Source: CAD feature listing. Evaluate the final solid. Frame: model axes, mm. Face numbers are marked on the shaded views. Give positions to 0.01 mm unless a question says otherwise; leave off trailing zeros. Loops run counter-clockwise (first coordinate to the right, second up) from the corner with the lowest first, then second, coordinate; pieces in that order, holes last. Notation, with made-up numbers: M -16,-36 L 3,-36 A10 cw 3,-23 Z; hole C 45.25,61 d9. An arc over 180 degrees is marked long. Put each result on its own line as item: value.
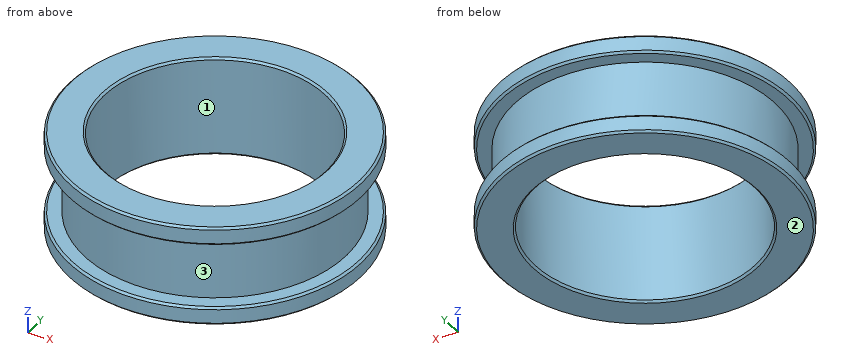
Autodesk Inventor part; units mm, degrees
ref_plane "Work Plane1" through (0, 0, 2.5) normal (0, 0, 1) x (1, 0, 0)
ref_plane "YZ Plane" through (0, 0, 0) normal (1, 0, 0) x (0, 1, 0)
ref_plane "XZ Plane" through (0, 0, 0) normal (0, 1, 0) x (-1, 0, 0)
sketch "Sketch1" plane through (0, 0, 0) normal (0, 0, 1) x (1, 0, 0)
  circle A0 centre (0, 0) radius 7.25
  dimension "d0" = 14.5
extrude "Extrusion1" add sketch "Sketch1" along normal blind 5
sketch "Sketch2" plane through (0, 0, 5) normal (0, 0, 1) x (1, 0, 0)
  circle A0 centre (0, 0) radius 5.5
  dimension "d3" = 11
extrude "Extrusion2" cut sketch "Sketch2" against normal through all
ref_plane "Work Plane1" through (0, 0, 2.5) normal (0, 0, 1) x (1, 0, 0)
sketch "Sketch3" plane through (0, 0, 2.5) normal (0, 0, 1) x (1, 0, 0)
  circle A0 centre (0, 0) radius 5.5
  circle A1 centre (0, 0) radius 6.5
  circle A2 centre (0, 0) radius 7.25
  dimension "d6" = 13
extrude "Extrusion3" cut sketch "Sketch3" along normal mid plane 3.2 contours A2
chamfer "Chamfer1" distance 0.1 angle 45 6 edges at (-7.25, 0, 4.1) (-7.25, 0, 0.9) (-7.25, 0, 0) (-7.25, 0, 5) (-5.5, 0, 0) (-5.5, 0, 5)
properties part number "roller" material "Aluminum 3004-H38"
1. Section query C-C (z = 4.45). Output: boundary loops of the cut face in (x, y), plus the area to 3 significant figures.
Found:
outline: C 0,0 d14.5; hole C 0,0 d11
area: 70.1 mm^2
2. Material intervals for line 1 (Y direction, x = 0, z = 4.55); line 2 (Y direction, x = 0, z = 3); line 3 (X direction, y = 4.5, z = 4), sorted ascending. Write a range as from..to.
Found:
line 1: -7.25..-5.5, 5.5..7.25
line 2: -6.5..-5.5, 5.5..6.5
line 3: -4.69..-3.16, 3.16..4.69
3. Contact query for flat-ended pins moving along their axis: P1, Ø1, axis at x = 4.5, z = 4.5, coming from the +Y side; P2, Ø1.5, axis at x = -1.5, z = 1, coming from the -Y side; P3, Ø2, axis at y = -2.5, z = 3, coming from the -X side. Output: stop coordinate, or through.
Found:
P1: y = 6.05
P2: y = -7.21
P3: x = -6.32
4. Section query D-D (z = 2.55). Output: boundary loops of the cut face in (x, y).
Found:
outline: C 0,0 d13; hole C 0,0 d11
5. Draft query along Y for the marked faces 1, 2 and 3. Return one class per face: pulls with the +Y half, pulls with the -Y half, needs draft (parallel to the pull), parting line crosses it, or undercut.
Found:
face 1: undercut
face 2: needs draft
face 3: parting line crosses it
6. Section query A-A (y = 0). Output: boundary loops of the cut face in (x, z).
Found:
outline: M -7.25,0.1 L -7.15,0 L -5.6,0 L -5.5,0.1 L -5.5,4.9 L -5.6,5 L -7.15,5 L -7.25,4.9 L -7.25,4.2 L -7.15,4.1 L -6.5,4.1 L -6.5,0.9 L -7.15,0.9 L -7.25,0.8 Z; M 5.5,0.1 L 5.6,0 L 7.15,0 L 7.25,0.1 L 7.25,0.8 L 7.15,0.9 L 6.5,0.9 L 6.5,4.1 L 7.15,4.1 L 7.25,4.2 L 7.25,4.9 L 7.15,5 L 5.6,5 L 5.5,4.9 Z
